Read the model definition and answer for the solid it produces. Units are mm, in the model's axes. Round coordinates to 2 decimals unless told otherwise and drop trailing zeros. Order: outer loops, then holes, each group sorted by start corner. A loop starts at its lowest first (then second) coordinate and runs counter-clockwise, first axis right, second up. Notation, with made-up numbers: (-29.75, -33) -> (-0.75, -33) arc R23 cw to (-0.75, -12) -> close; hole circle Ø10 at (39, -38). An arc over 180 degrees is marked (long way). One line per item, written item: value. Start each with the question number.
1. Consider line 1 (Y direction, x = 45, z = 4); line 2 (Y direction, x = 25, z = 3.75); line 3 (X direction, y = 25, z = 2). Determine where each line is inside the solid, lowest interval first.
2. A flat-ended cylindrical pin translates along its axis: pin 1 Ø2.5 at (x, y) = (5, 5) entering from -Z. Find the tip coordinate at first contact, or state that the pin passes through.
3. Section D-D (y = 25) is taken. Give the vertices of the cut face in (x, z), then the cut area to 3 significant figures.
4. Section A-A (y = 5) is taken. Give the vertices of the cut face in (x, z), then the cut area to 3 significant figures.
5. The mould has two halves that part along Y. Classify faces 1 (the face through (25, 27.5, 5)), 2 (the face through (25, 0, 5)), 3 (the face through (19, 25, 0)): released by +Y, released by -Y, zero draft, split by the parting line, or undercut.
6. Section B-B (x = 25) is taken. Give the vertices of the cut face in (y, z), then the cut area to 3 significant figures.
from build123d import *

# Parameters (mm, degrees)
IZIM1_W                     = 50
IZIM1_H                     = 50
IZIM1_R                     = 2
Y_KSEKLIK_EKSTR_ZYON1_DEPTH = 10


with BuildPart() as part:
    # Çizim1 → Yükseklik-Ekstrüzyon1 (new body)
    with BuildSketch(Plane.XY):
        with Locations((25, 25)):
            Rectangle(IZIM1_W, IZIM1_H)
        with Locations((5, 45)):
            Circle(IZIM1_R, mode=Mode.SUBTRACT)
        with Locations((45, 45)):
            Circle(IZIM1_R, mode=Mode.SUBTRACT)
        with Locations((45, 5)):
            Circle(IZIM1_R, mode=Mode.SUBTRACT)
        with Locations((5, 5)):
            Circle(IZIM1_R, mode=Mode.SUBTRACT)
        with BuildLine():
            Line((22.845934077, 27.5), (27.154065923, 27.5))
            ThreePointArc((27.154065923, 27.5), (25, 21.7), (22.845934077, 27.5))
        make_face(mode=Mode.SUBTRACT)
    extrude(amount=Y_KSEKLIK_EKSTR_ZYON1_DEPTH)


solid = part.part
Answer:
1. line 1: 0 to 3, 7 to 43, 47 to 50
1. line 2: 0 to 21.7, 27.5 to 50
1. line 3: 0 to 21.7, 28.3 to 50
2. pin 1: through
3. outline: (0, 0) -> (21.7, 0) -> (21.7, 10) -> (0, 10) -> close; (28.3, 0) -> (50, 0) -> (50, 10) -> (28.3, 10) -> close
3. area: 434 mm^2
4. outline: (0, 0) -> (3, 0) -> (3, 10) -> (0, 10) -> close; (7, 0) -> (43, 0) -> (43, 10) -> (7, 10) -> close; (47, 0) -> (50, 0) -> (50, 10) -> (47, 10) -> close
4. area: 420 mm^2
5. face 1: undercut
5. face 2: released by -Y
5. face 3: zero draft
6. outline: (0, 0) -> (21.7, 0) -> (21.7, 10) -> (0, 10) -> close; (27.5, 0) -> (50, 0) -> (50, 10) -> (27.5, 10) -> close
6. area: 442 mm^2
